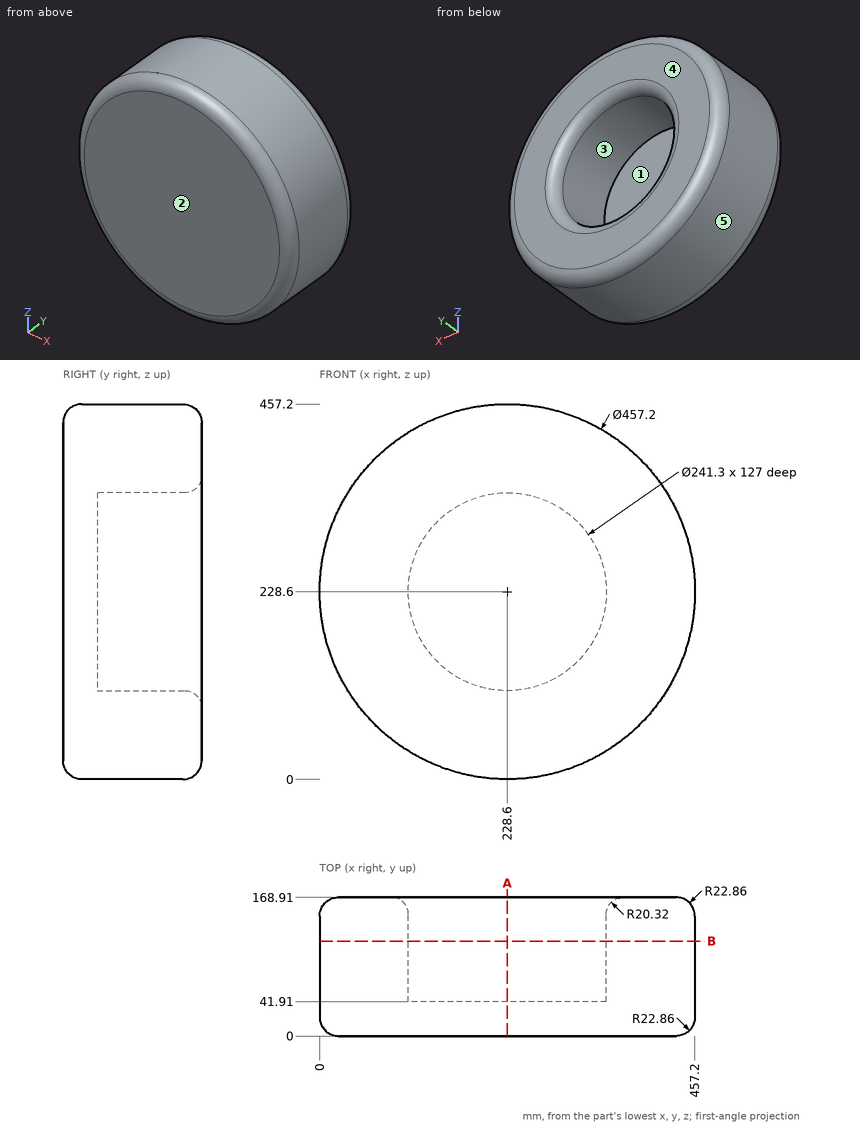
Drawing for the job (mm, zero at the part's lowest x, y, z). A direction names the side the tool comes from. Round coordinates to 2 decimals unless told otherwise and drop trailing zeros. Order: outer loops, then holes, each group sorted by start corner. A loop starts at its lowest first (then second) coordinate and runs counter-clockwise, first axis right, second up. Notation, with made-up numbers: M 30.25,57.25 L 85.25,57.25 A23 ccw 85.25,88.25 Z; hole C 43,-27 d9. An arc over 180 degrees is marked long. Use one line per item in the form item = value.
Q1. Which spindle directions (+Z, -Z, +X, -X, +Y, -Y) get a long thin tool onto all of the face, cutting with end or side? Do the marked faces 1 and 2. Say none if no direction does.
Recorded:
face_1 = +Y
face_2 = +Z, -Z, +X, -X, -Y
Q2. Saw through at B-B on y = 115.5. Give the cut face in (x, z), then the cut area to 3 significant figures.
Recorded:
outline = C 228.6,228.6 d457.2; hole C 228.6,228.6 d241.3
area = 118,000 mm^2
Q3. Saw through at A-A on x = 228.6. Give the cut face in (y, z).
Recorded:
outline = M 0,22.86 A22.86 ccw 22.86,0 L 146.05,0 A22.86 ccw 168.91,22.86 L 168.91,87.63 A20.32 ccw 148.59,107.95 L 41.91,107.95 L 41.91,349.25 L 148.59,349.25 A20.32 ccw 168.91,369.57 L 168.91,434.34 A22.86 ccw 146.05,457.2 L 22.86,457.2 A22.86 ccw 0,434.34 Z
Q4. Probe L1, parallel to X at y = 89.5, z = 228.6; L2, parallel to Y at x = 353, z = 293. List the from-to ranges inside material, lowest first.
Recorded:
L1 = 0 to 107.95, 349.25 to 457.2
L2 = 0 to 168.89
Q5. Two-plate mould, pull along Z, no slides. Class the marked faces 3, 4 and 5: +Z half, -Z half, draft (parallel to the pull), parting line (faces both ways), or undercut.
Recorded:
face_3 = undercut
face_4 = draft
face_5 = parting line
Q6. Flat gauge pins, fed straight in: P1, Ø4, axis at y = 152, z = 198, coming from the +X side; P2, Ø12, axis at x = 166.5, z = 298.5, coming from the +Y side; P3, Ø1.5, axis at x = 146, y = 102.5, coming from the +Z side. Where does each tip first touch, or does it go through?
Recorded:
P1 = 454.88
P2 = 41.91
P3 = 442.04
